Source: CAD feature listing. Evaluate the final solid. Frame: model axes, mm. A direction names the side the tool comes from. Round coordinates to 2 decimals unless told otherwise and drop trailing zeros. Loops run counter-clockwise (first coordinate to the right, second up) from the corner with the lowest first, then second, coordinate; pieces in that order, holes last. Notation, with made-up numbers: (81, 75.25) -> (127, 75.25) arc R29 cw to (127, 96.25) -> close; hole circle Ø5 at (33, 36). An arc over 180 degrees is marked (long way). Put each result on its own line as item: value. Start each with the question number.
1. Cut plane B-B (y = 31.5). Return the cut outline in (x, z).
2. Contact query for flat-ended pins moving along their axis: pin 1 (1.5 mm diameter, centred on x = 35.5, z = 5, fed in from +Y); pin 2 (5 mm diameter, centred on x = -14.5, y = 37, fed in from -Z); pin 3 (2 mm diameter, centred on x = -36, z = 5, fed in from -Y); pin 4 (3 mm diameter, centred on y = 20, z = 2.5, fed in from -X). Output: stop coordinate, or through.
3. Material intervals for L1, parallel to Y at x = 19.5, z = 1.5; L2, parallel to X at y = -22.5, z = 1.5; L3, parallel to Y at x = -4, z = 7.5, sorted ascending.
4. Draft query along X for faces 3 (the flat face through (0, 25, 10)), 4 (the flat face through (-24.6, 15.12, 6.04)), 5 (the flat face through (15.3, 4.73, 8.23)). Return one class per face: pulls with the +X half, pulls with the -X half, needs draft (parallel to the pull), parting line crosses it, or undercut.
5. Cut plane C-C (x = -41.5). Return the cut outline in (y, z), then the cut area to 3 significant figures.
6. Cut plane A-A (z = 2). Return the cut outline in (x, y), then the cut area to 3 significant figures.
7. Set-up query: faces 1 (the flat face through (-11.751, 10.887, 8.226)), 2 (the flat face through (21, -13, 10)). Return all of +Z, -Z, +X, -X, +Y, -Y with unobstructed straight access to the full face (end or side cutting, diameter ignored); none if empty.
```python
from build123d import *

# Parameters (mm, degrees)
F1_DEPTH  = 10
F3_DEPTH  = 29
F5_DEPTH  = 29
F7_DEPTH  = 29
F8_W      = 7
F8_H      = 3.5
F9_DEPTH  = 29
F10_W     = 7
F10_H     = 3.5
F11_DEPTH = 29
F12_W     = 7
F12_H     = 3.5
F13_DEPTH = 29


with BuildPart() as f1:
    # F0 (on Top) → F1 (new body)
    with BuildSketch(Plane.XY):
        Polygon((49.9008693401, -29.0385359899), (0.1976751859, 57.7346885144), (-50.098544526, -28.6961525245), align=None)
    extrude(amount=F1_DEPTH)

    # F2 (on face) → F3 (cut)
    with BuildSketch(Plane(origin=(-0.0988375929, -28.8673442572, 0), x_dir=(0.9999941387, -0.0034238347, 0), z_dir=(-0.0034238347, -0.9999941387, 0))):
        with BuildLine():
            Line((-5, 0), (5, 0))
            ThreePointArc((5, 0), (0, 5), (-5, 0))
        make_face()
    extrude(amount=-F3_DEPTH, mode=Mode.SUBTRACT)

    # F4 (on face) → F5 (cut)
    with BuildSketch(Plane(origin=(-24.9504346701, 14.5192679949, 0), x_dir=(-0.5029621971, -0.8643084104, 0), z_dir=(-0.8643084104, 0.5029621971, 0))):
        with BuildLine():
            Line((-5, 0), (5, 0))
            ThreePointArc((5, 0), (0, 5), (-5, 0))
        make_face()
    extrude(amount=-F5_DEPTH, mode=Mode.SUBTRACT)

    # F6 (on face) → F7 (cut)
    with BuildSketch(Plane(origin=(25.049272263, 14.3480762623, 0), x_dir=(-0.4970319415, 0.867732245, 0), z_dir=(0.867732245, 0.4970319415, 0))):
        with BuildLine():
            Line((-5, 0), (5, 0))
            ThreePointArc((5, 0), (0, 5), (-5, 0))
        make_face()
    extrude(amount=-F7_DEPTH, mode=Mode.SUBTRACT)

    # F8 (on face) → F9 (cut)
    with BuildSketch(Plane(origin=(25.049272263, 14.3480762623, 0), x_dir=(-0.4970319415, 0.867732245, 0), z_dir=(0.867732245, 0.4970319415, 0))):
        with Locations((0, 8.25)):
            Rectangle(F8_W, F8_H)
    extrude(amount=-F9_DEPTH, mode=Mode.SUBTRACT)

    # F10 (on face) → F11 (cut)
    with BuildSketch(Plane(origin=(-24.9504346701, 14.5192679949, 0), x_dir=(-0.5029621971, -0.8643084104, 0), z_dir=(-0.8643084104, 0.5029621971, 0))):
        with Locations((0, 8.25)):
            Rectangle(F10_W, F10_H)
    extrude(amount=-F11_DEPTH, mode=Mode.SUBTRACT)

    # F12 (on face) → F13 (cut)
    with BuildSketch(Plane(origin=(-0.0988375929, -28.8673442572, 0), x_dir=(0.9999941387, -0.0034238347, 0), z_dir=(-0.0034238347, -0.9999941387, 0))):
        with Locations((0, 8.25)):
            Rectangle(F12_W, F12_H)
    extrude(amount=-F13_DEPTH, mode=Mode.SUBTRACT)


solid = f1.part
```
Solution:
1. outline: (-15.07, 0) -> (15.22, 0) -> (15.22, 10) -> (-15.07, 10) -> close
2. pin 1: stops at y = -2.59
2. pin 2: stops at z = 0
2. pin 3: stops at y = -28.75
2. pin 4: stops at x = -22.63
3. L1: y = -28.93 to 5.67, 16.67 to 24.04
3. L2: x = -46.49 to -4.85, 4.69 to 46.16
3. L3: y = -28.85 to -1.72, 6.38 to 50.52
4. face 3: needs draft
4. face 4: pulls with the -X half
4. face 5: undercut
5. outline: (-28.73, 0) -> (-13.92, 0) -> (-13.92, 10) -> (-28.73, 10) -> close
5. area: 148 mm^2
6. outline: (-50.1, -28.7) -> (-4.68, -28.85) -> (-4.59, -2.63) -> (-27.26, 10.56) -> close; (-22.65, 18.48) -> (0.02, 5.29) -> (22.77, 18.32) -> (0.2, 57.73) -> close; (4.48, -28.88) -> (49.9, -29.04) -> (27.33, 10.37) -> (4.57, -2.66) -> close
6. area: 3,570 mm^2
7. face 1: +Z
7. face 2: +Z, +X, -X, +Y, -Y
